```python
from build123d import *

# Parameters (mm, degrees)
SKETCH1_R               = 7.5
BOSS_EXTRUDE1_DEPTH     = 13
BOSS_EXTRUDE2_DEPTH     = 13
BOSS_EXTRUDE3_DEPTH     = 35
BOSS_EXTRUDE4_DEPTH     = 8
CUT_EXTRUDE3_DEPTH      = 6
CUT_EXTRUDE3_DEPTH_BACK = 6
BOSS_EXTRUDE5_DEPTH     = 53
SKETCH11_R              = 2
CUT_EXTRUDE4_DEPTH      = 0.1
SKETCH12_R              = 1
CUT_EXTRUDE5_DEPTH      = 52
SKETCH16_R              = 5.5
CUT_EXTRUDE8_DEPTH      = 0.1
SKETCH17_R              = 2.5
CUT_EXTRUDE9_DEPTH      = 20.1
CUT_EXTRUDE10_DEPTH     = 11
CUT_EXTRUDE11_DEPTH     = 25
CUT_EXTRUDE12_DEPTH     = 10
FILLET1_R               = 1


with BuildPart() as part:
    # Sketch1 → Boss-Extrude1 (new body)
    with BuildSketch(Plane(origin=(0, 0, 0), x_dir=(1, 0, 0), z_dir=(0, 1, 0))):
        with BuildLine():
            Line((-15.000119656, -22.499966246), (15.000119656, -22.499966246))
            Line((15.000119656, -22.499966246), (15.000119656, -14.499966246))
            Line((15.000119656, -14.499966246), (10.105611377, 2.850722488))
            ThreePointArc((10.105611377, 2.850722488), (0, 10.5), (-10.105611377, 2.850722488))
            Line((-10.105611377, 2.850722488), (-15.000119656, -14.499966246))
            Line((-15.000119656, -14.499966246), (-15.000119656, -22.499966246))
        make_face()
        with Locations(Location((0, 0, 0), (0, 0, 90))):
            Circle(SKETCH1_R, mode=Mode.SUBTRACT)
    extrude(amount=BOSS_EXTRUDE1_DEPTH)

    # Sketch2 → Boss-Extrude2 (add)
    with BuildSketch(Plane(origin=(0, 0, 0), x_dir=(1, 0, 0), z_dir=(0, 1, 0))):
        Polygon((-15.000119656, -22.499966246), (-15.000119656, -30.499966246), (14.999880344, -30.499966246), (15.000119656, -22.499966246), align=None)
    extrude(amount=BOSS_EXTRUDE2_DEPTH)

    # Sketch3 → Boss-Extrude3 (add)
    with BuildSketch(Plane.XZ):
        Polygon((-15.000119656, 30.499966246), (14.999880344, 30.499966246), (15.000119656, 22.499966246), (-15.000119656, 22.499966246), align=None)
    extrude(amount=BOSS_EXTRUDE3_DEPTH)

    # Sketch4 → Boss-Extrude4 (add)
    with BuildSketch(Plane.XY.offset(30.499966246)):
        with BuildLine():
            Line((14.999880344, -35), (14.999880344, 13))
            ThreePointArc((14.999880344, 13), (20.461578839, -11), (14.999880344, -35))
        make_face()
        with BuildLine():
            Line((-15.000119656, -35), (-15.000119656, 13))
            ThreePointArc((-15.000119656, 13), (-20.461818151, -11), (-15.000119656, -35))
        make_face()
    extrude(amount=-BOSS_EXTRUDE4_DEPTH)

    # Sketch9 → Cut-Extrude3 (cut, two sides: drawn at the far end of the back side and taken through both)
    with BuildSketch(Plane.XY.offset(22.5).offset(-CUT_EXTRUDE3_DEPTH_BACK)):
        with BuildLine():
            Line((-13.33053559, -32), (11.997996308, -32))
            Line((11.997996308, -32), (13.330296278, -32))
            ThreePointArc((13.330296278, -32), (17.049056164, -17.737940448), (16.879854834, -3))
            Line((16.879854834, -3), (15, -3))
            Line((15, -3), (-16.880094146, -3))
            ThreePointArc((-16.880094146, -3), (-17.049295477, -17.737940448), (-13.33053559, -32))
        make_face()
    extrude(amount=CUT_EXTRUDE3_DEPTH + CUT_EXTRUDE3_DEPTH_BACK, mode=Mode.SUBTRACT)

    # Sketch10 → Boss-Extrude5 (add)
    with BuildSketch(Plane.XY.offset(30.499966246)):
        with BuildLine():
            Line((-3.500119656, -28.5), (-0.750119656, -28.5))
            Line((-0.750119656, -28.5), (-0.750119656, -25.5))
            Line((-0.750119656, -25.5), (-0.000119656, -25.5))
            Line((-0.000119656, -25.5), (0.749880344, -25.5))
            Line((0.749880344, -25.5), (0.749880344, -28.5))
            Line((0.749880344, -28.5), (3.499880344, -28.5))
            Line((3.499880344, -28.5), (3.499880344, -31.5))
            ThreePointArc((3.499880344, -31.5), (-0.000119656, -35), (-3.500119656, -31.5))
            Line((-3.500119656, -31.5), (-3.500119656, -28.5))
        make_face()
        with BuildLine():
            Line((0.749880344, 6.5), (3.499880344, 6.5))
            Line((3.499880344, 6.5), (3.499880344, 9.5))
            ThreePointArc((3.499880344, 9.5), (-0.000119656, 13), (-3.500119656, 9.5))
            Line((-3.500119656, 9.5), (-3.500119656, 6.5))
            Line((-3.500119656, 6.5), (-0.750119656, 6.5))
            Line((-0.750119656, 6.5), (-0.750119656, 3.5))
            Line((-0.750119656, 3.5), (-0.000119656, 3.5))
            Line((-0.000119656, 3.5), (0.749880344, 3.5))
            Line((0.749880344, 3.5), (0.749880344, 6.5))
        make_face()
    extrude(amount=BOSS_EXTRUDE5_DEPTH)

    # Sketch11 → Cut-Extrude4 (cut)
    with BuildSketch(Plane.XY.offset(83.499966246)):
        with Locations((-0.000119656, -31.5)):
            Circle(SKETCH11_R)
        with Locations((-0.000119656, 9.5)):
            Circle(SKETCH11_R)
    extrude(amount=-CUT_EXTRUDE4_DEPTH, mode=Mode.SUBTRACT)

    # Sketch12 → Cut-Extrude5 (cut)
    with BuildSketch(Plane.XY.offset(83.399966246)):
        with Locations((-0.000119656, -31.5)):
            Circle(SKETCH12_R)
        with Locations((-0.000119656, 9.5)):
            Circle(SKETCH12_R)
    extrude(amount=-CUT_EXTRUDE5_DEPTH, mode=Mode.SUBTRACT)

    # Sketch16 → Cut-Extrude8 (cut)
    with BuildSketch(Plane(origin=(10.105611377, 0, -2.850722488), x_dir=(-0.27149737978458055, 0, -0.9624391787381202), z_dir=(0.9624391787381201, 0, -0.2714973797845805))):
        with Locations((-6, 6.5)):
            Circle(SKETCH16_R)
    extrude(amount=-CUT_EXTRUDE8_DEPTH, mode=Mode.SUBTRACT)

    # Sketch17 → Cut-Extrude9 (cut)
    with BuildSketch(Plane(origin=(10.009367459, 0, -2.82357275), x_dir=(-0.2714973797845806, 0, -0.9624391787381202), z_dir=(0.9624391787381201, 0, -0.27149737978458055))):
        with Locations((-6, 6.5)):
            Circle(SKETCH17_R)
    extrude(amount=-CUT_EXTRUDE9_DEPTH, mode=Mode.SUBTRACT)

    # Sketch18 → Cut-Extrude10 (cut)
    with BuildSketch(Plane.XZ):
        with BuildLine():
            Line((-8.45474492, 13.294804883), (-8.86199099, 11.851146114))
            ThreePointArc((-8.86199099, 11.851146114), (-12.563800666, 9.778320718), (-10.490975269, 6.076511042))
            Line((-10.490975269, 6.076511042), (-10.898221339, 4.632852274))
            Line((-10.898221339, 4.632852274), (-7.048464624, 3.546862755))
            Line((-7.048464624, 3.546862755), (-4.604988206, 12.208815363))
            Line((-4.604988206, 12.208815363), (-8.45474492, 13.294804883))
        make_face()
    extrude(amount=-CUT_EXTRUDE10_DEPTH, mode=Mode.SUBTRACT)

    # Sketch19 → Cut-Extrude11 (cut)
    with BuildSketch(Plane.XZ):
        Polygon((16.189167047, 14.774953484), (16.896273828, 15.482060265), (15.482060265, 16.896273828), (14.774953484, 16.189167047), (14.067846703, 15.482060265), (3.042893219, 4.457106781), (4.457106781, 3.042893219), (15.482060265, 14.067846703), align=None)
    extrude(amount=-CUT_EXTRUDE11_DEPTH, mode=Mode.SUBTRACT)

    # Sketch20 → Cut-Extrude12 (cut)
    with BuildSketch(Plane.XZ):
        Polygon((-12.998307469, 20.504333218), (-12.998307469, 19.504333218), (4.548842229, 8.791482916), (12.171692531, 16.414333218), (12.171692531, 20.504333218), align=None)
    extrude(amount=-CUT_EXTRUDE12_DEPTH, mode=Mode.SUBTRACT)

    # Fillet1
    fillet1_edges = [part.edges().sort_by_distance(p)[0] for p in [
        (14.640950567, 6.5, 13.226737005),
        (12.171692531, 5, 16.414333218),
        (4.548842229, 5, 8.791482916),
        (-13.33053559, -32, 25.499983123),
        (-17.049295477, -17.737940448, 28.5),
        (-16.880094146, -3, 25.499983123),
        (-0.000119656, -3, 28.5),
        (16.879854834, -3, 25.499983123),
        (13.330296278, -32, 25.499983123),
        (-0.000119656, -32, 28.5),
        (17.049056164, -17.737940448, 28.5),
    ]]
    fillet(fillet1_edges, radius=FILLET1_R)


solid = part.part
```
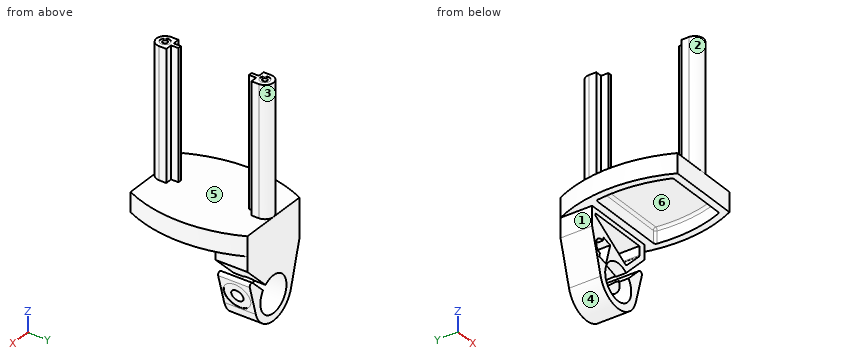
Verification items for the finished model (mm, model axes). Face numbers are marked on the shaded views. A direction names the side the tool comes from. Coordinates: 2 decimals unless noted, no trailing zeros. Loops run counter-clockwise (first coordinate to the right, second up) from the corner with the lowest first, then second, coordinate; pieces in that order, holes last. Notation, with made-up numbers: (61.25, 43) -> (112.25, 43) arc R26 ccw to (112.25, 67) -> close; hole circle Ø4 at (43, -24). An arc over 180 degrees is marked (long way). Answer in a Markdown table with one row per item.
1) Depth check by flat-ended pin: P1, Ø19.5, axis at x = 0, z = 0, coming from the +Y side; P2, Ø0.9, axis at y = -29.5, z = 46, coming from the -X side; P3, Ø0.6, axis at x = 0, y = -31, coming from the +Z side; P4, Ø0.8, axis at x = 3, z = 67, coming from the +Y side. Enter the tip coordinate at first touch or a pass-through.
The answers:
| item | result |
|---|---|
| P1 | stops at y = 13 |
| P2 | stops at x = -3.5 |
| P3 | stops at z = 31.4 |
| P4 | stops at y = 11.84 |
2) Draft check along X on the marked faces 4, 5 and 6. Enter one of: released by +X, released by -X, zero draft, split by the parting line, or undercut.
The answers:
| item | result |
|---|---|
| face 4 | split by the parting line |
| face 5 | zero draft |
| face 6 | undercut |
3) Scan lines: line 1 along Z through (x, y) = (0, 5.25); line 2 along Z through (x, y) = (0, 4); line 3 along Z through (x, y) = (1, -4). Record each from-to range of solid material in increasing order. Write a range as from..to.
The answers:
| item | result |
|---|---|
| line 1 | z = -10.5..-7.5, 8.48..11.57, 20.5..83.5 |
| line 2 | z = -10.5..-7.5, 7.5..11.57, 20.5..83.5 |
| line 3 | z = 28.5..30.5 |
4) Section check A-A (z = 54). Record the cut outline in (x, y).
The answers:
| item | result |
|---|---|
| outline | (-3.5, -31.5) arc R3.5 ccw to (3.5, -31.5) -> (3.5, -28.5) -> (0.75, -28.5) -> (0.75, -25.5) -> (-0.75, -25.5) -> (-0.75, -28.5) -> (-3.5, -28.5) -> close; (-3.5, 6.5) -> (-0.75, 6.5) -> (-0.75, 3.5) -> (0.75, 3.5) -> (0.75, 6.5) -> (3.5, 6.5) -> (3.5, 9.5) arc R3.5 ccw to (-3.5, 9.5) -> close; hole circle Ø2 at (0, -31.5); hole circle Ø2 at (0, 9.5) |
5) Access from +Z, -Z, +X, -X, +Y, -Y to the whole of each face (thin tool, end or side, straight path). Record for the marked faces 1, 2 and 3.
The answers:
| item | result |
|---|---|
| face 1 | -Z, -X, +Y, -Y |
| face 2 | +Z, -Y |
| face 3 | +Z, +Y |
